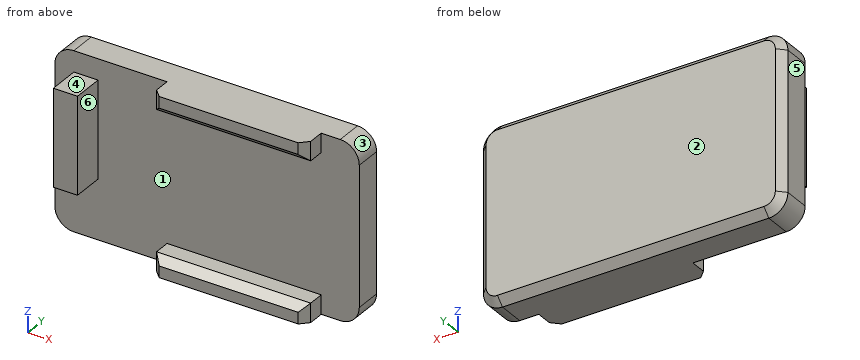
```python
from build123d import *

# Parameters (mm, degrees)
SKETCH_1_W      = 32
SKETCH_1_H      = 18.6
EXTRUDE_1_DEPTH = 3.6
SKETCH_2_W      = 2.54
SKETCH_2_H      = 10.16
EXTRUDE_2_DEPTH = 3.3
SKETCH_3_W      = 16.2
SKETCH_3_H      = 2
EXTRUDE_3_DEPTH = 2.5
FILLET_1_R      = 2
CHAMFER_1_SIZE  = 0.8
CHAMFER_2_SIZE  = 0.8


with BuildPart() as part:
    # 草图1 → 凸台-拉伸1 (new body)
    with BuildSketch(Plane(origin=(0, 0, 0), x_dir=(1, 0, 0), z_dir=(0, 1, 0))):
        with Locations((78.299519248, 9.3)):
            Rectangle(SKETCH_1_W, SKETCH_1_H)
    extrude(amount=EXTRUDE_1_DEPTH)

    # 草图2 → 凸台-拉伸2 (add)
    with BuildSketch(Plane.XZ):
        with Locations((65.569519248, -7.28)):
            Rectangle(SKETCH_2_W, SKETCH_2_H)
    extrude(amount=EXTRUDE_2_DEPTH)

    # 草图3 → 凸台-拉伸3 (add)
    with BuildSketch(Plane.XZ):
        with Locations((82.199519248, -17.6)):
            Rectangle(SKETCH_3_W, SKETCH_3_H)
        with Locations((82.199519248, -1)):
            Rectangle(SKETCH_3_W, SKETCH_3_H)
    extrude(amount=EXTRUDE_3_DEPTH)

    # 圆角1
    fillet_1_edges = [part.edges().sort_by_distance(p)[0] for p in [
        (62.299519248, 1.8, -18.6),
        (94.299519248, 1.8, -18.6),
        (94.299519248, 1.8, 0),
        (62.299519248, 1.8, 0),
    ]]
    fillet(fillet_1_edges, radius=FILLET_1_R)

    # 倒角1
    chamfer_1_edges = [part.edges().sort_by_distance(p)[0] for p in [
        (62.299519248, 3.6, -9.3),
        (78.299519248, 3.6, -18.6),
        (78.299519248, 3.6, 0),
        (94.299519248, 3.6, -9.3),
        (62.885305686, 3.6, -0.585786438),
        (93.71373281, 3.6, -0.585786438),
        (93.71373281, 3.6, -18.014213562),
        (62.885305686, 3.6, -18.014213562),
    ]]
    chamfer(chamfer_1_edges, length=CHAMFER_1_SIZE)

    # 倒角2
    chamfer_2_edges = [part.edges().sort_by_distance(p)[0] for p in [
        (90.299519248, -2.5, -17.6),
        (82.199519248, -2.5, -16.6),
        (74.099519248, -2.5, -17.6),
        (82.199519248, -2.5, -2),
        (90.299519248, -2.5, -1),
        (74.099519248, -2.5, -1),
    ]]
    chamfer(chamfer_2_edges, length=CHAMFER_2_SIZE)


solid = part.part
```
Geometry check sheet. Reference: the model listing, model coordinates, mm. Face numbers are marked on the shaded views. A direction names the side the tool comes from. Coordinates: 2 decimals unless noted, no trailing zeros. Write each loop counter-clockwise with the first axis right and the second up, starting at its lowest first coordinate (ties: lowest second). Pieces come first, ordered by that corner, then holes. Notation, with made-up numbers: (82.5, 45) -> (90.5, 45) arc R16 cw to (90.5, 56) -> close; hole circle Ø1 at (70, 36). An arc over 180 degrees is marked (long way). Use CSV: the item, a comma, the result in double quotes. Start each with the question number.
Item 1: Cross-section at A-A, the plane y = -0.75. Record the cut outline in (x, z), plus the area to 3 significant figures.
Item 2: Cross-section at B-B, the plane z = -5.75. Record the cut outline in (x, y), plus the area to 3 significant figures.
Item 3: Cross-section at C-C, the plane x = 73.5. Record the cut outline in (y, z).
Item 4: Cross-section at D-D, the plane y = 3.25. Record the cut outline in (x, z), plus the area to 3 significant figures.
Item 5: Thickness scan on line 1 (Z direction, x = 81, y = -0.25); line 2 (Y direction, x = 81, z = -17.5); line 3 (X direction, y = -2, z = -5.5). Record the ranges inside material, lowest first.
Item 6: Depth check by flat-ended pin: pin 1 Ø0.5 at (y, z) = (-1, -17.5) entering from -X; pin 2 Ø9.5 at (x, z) = (80.5, -5) entering from -Y; pin 3 Ø1.4 at (y, z) = (-1, -0.5) entering from +X. Enter the tip coordinate at first touch or a pass-through.
Item 7: Set-up check for the marked faces 4, 5 and 6: record each of +Z, -Z, +X, -X, +Y, -Y from which the full face is reachable in a straight line by a thin tool's end or side.
Item 8: Mould release check, pull along Z, two halves, no side actions. Record for the marked faces 1, 2 and 3: released by +Z, released by -Z, zero draft, split by the parting line, or undercut.
Answers:
1,outline,"(64.3, -12.36) -> (66.84, -12.36) -> (66.84, -2.2) -> (64.3, -2.2) -> close; (74.1, -18.6) -> (90.3, -18.6) -> (90.3, -16.6) -> (74.1, -16.6) -> close; (74.1, -2) -> (90.3, -2) -> (90.3, 0) -> (74.1, 0) -> close"
1,area,"90.6 mm^2"
2,outline,"(62.3, 0) -> (64.3, 0) -> (64.3, -3.3) -> (66.84, -3.3) -> (66.84, 0) -> (94.3, 0) -> (94.3, 2.8) -> (93.5, 3.6) -> (63.1, 3.6) -> (62.3, 2.8) -> close"
2,area,"123 mm^2"
3,outline,"(0, -18.6) -> (2.8, -18.6) -> (3.6, -17.8) -> (3.6, -0.8) -> (2.8, 0) -> (0, 0) -> close"
4,outline,"(62.75, -16.6) arc R1.55 ccw to (64.3, -18.15) -> (92.3, -18.15) arc R1.55 ccw to (93.85, -16.6) -> (93.85, -2) arc R1.55 ccw to (92.3, -0.45) -> (64.3, -0.45) arc R1.55 ccw to (62.75, -2) -> close"
4,area,"548 mm^2"
5,line 1,"-18.6 to -16.6, -2 to 0"
5,line 2,"-2.5 to 3.6"
5,line 3,"64.3 to 66.84"
6,pin 1,"x = 74.1"
6,pin 2,"y = -2.5"
6,pin 3,"x = 90.3"
7,face 4,"+Z, +X, -X, -Y"
7,face 5,"+Z, -Z, -X, +Y, -Y"
7,face 6,"+Z, -Z, +X, -Y"
8,face 1,"undercut"
8,face 2,"zero draft"
8,face 3,"released by +Z"
